Geometry: final body of the model. Coordinates: model frame, mm. Give positions to 0.01 mm unless a question says otherwise; leave off trailing zeros. Loops run counter-clockwise (first coordinate to the right, second up) from the corner with the lowest first, then second, coordinate; pieces in that order, holes last. Notation, with made-up numbers: (-21.5, 32) - (1.5, 32) arc R27 cw to (1.5, 51) - close; hole circle Ø8 at (36, 86.25). An arc over 180 degrees is marked (long way). Use CSV: the item, a comma, the result in double quotes. Start each with the question number.
```python
from build123d import *

# Parameters (mm, degrees)
SKETCH1_W             = 560
SKETCH1_H             = 560
BOSS_EXTRUDE1_DEPTH   = 3
F_4_0MM_DOWEL_HOLE1_D = 4
SKETCH5_R             = 5.15
CUT_EXTRUDE1_DEPTH    = 10
SKETCH6_R             = 7.5
CUT_EXTRUDE2_DEPTH    = 10


with BuildPart() as part:
    # Sketch1 → Boss-Extrude1 (new body)
    with BuildSketch(Plane(origin=(0, 0, 0), x_dir=(1, 0, 0), z_dir=(0, 1, 0))):
        with Locations((280, 280)):
            Rectangle(SKETCH1_W, SKETCH1_H)
    extrude(amount=BOSS_EXTRUDE1_DEPTH)

    # Ø4.0mm Dowel Hole1 (through all)
    with Locations(Plane(origin=(0, 3, 0), x_dir=(1, 0, 0), z_dir=(0, 1, 0))):
        with Locations((159, 159), (401, 159), (401, 401), (159, 401)):
            Hole(F_4_0MM_DOWEL_HOLE1_D / 2)

    # Sketch5 → Cut-Extrude1 (cut)
    with BuildSketch(Plane(origin=(0, 3, 0), x_dir=(1, 0, 0), z_dir=(0, 1, 0))):
        with Locations(Location((41, 280, 0), (0, 0, 270))):
            Circle(SKETCH5_R)
        with Locations(Location((519, 280, 0), (0, 0, 270))):
            Circle(SKETCH5_R)
    extrude(amount=-CUT_EXTRUDE1_DEPTH, mode=Mode.SUBTRACT)

    # Sketch6 → Cut-Extrude2 (cut)
    with BuildSketch(Plane(origin=(0, 3, 0), x_dir=(1, 0, 0), z_dir=(0, 1, 0))):
        with Locations(Location((495, 15, 0), (0, 0, 270))):
            Circle(SKETCH6_R)
        with Locations(Location((65, 15, 0), (0, 0, 270))):
            Circle(SKETCH6_R)
        with Locations(Location((495, 545, 0), (0, 0, 90))):
            Circle(SKETCH6_R)
        with Locations(Location((65, 545, 0), (0, 0, 90))):
            Circle(SKETCH6_R)
    extrude(amount=-CUT_EXTRUDE2_DEPTH, mode=Mode.SUBTRACT)


solid = part.part
```
Item 1: Mould query, pull axis X, two halves, no side actions, for faces 1 (the cylindrical face through (502.436, 1.521, -15.976)), 2 (the flat face through (276, 3, -284)). Classes: pulls with the +X half, pulls with the -X half, needs draft (parallel to the pull), parting line crosses it, or undercut.
Item 2: Section A-A (z = -15). Output: boundary loops of the cut face in (x, y), plus the area to 3 significant figures.
Item 3: Ray query, probe 1 along X at (y, z) = (1.3, -545); probe 2 along X at (y, z) = (1.45, -280); probe 3 along Z at (x, y) = (401, 2.1). Return the intervals inside material, ascending.
Outcome:
1,face 1,"undercut"
1,face 2,"needs draft"
2,outline,"(0, 0) - (57.5, 0) - (57.5, 3) - (0, 3) - close; (72.5, 0) - (487.5, 0) - (487.5, 3) - (72.5, 3) - close; (502.5, 0) - (560, 0) - (560, 3) - (502.5, 3) - close"
2,area,"1,590 mm2"
3,probe 1,"x = 0 to 57.5, 72.5 to 487.5, 502.5 to 560"
3,probe 2,"x = 0 to 35.85, 46.15 to 513.85, 524.15 to 560"
3,probe 3,"z = -560 to -403, -399 to -161, -157 to 0"
